CAD build for the part. Positions are in the model's coordinates, mm. A direction names the side the tool comes from. Round coordinates to 2 decimals unless told otherwise and drop trailing zeros. Order: outer loops, then holes, each group sorted by start corner. A loop starts at its lowest first (then second) coordinate and runs counter-clockwise, first axis right, second up. Notation, with made-up numbers: M 41,47 L 55,47 A18 cw 55,74 Z; hole C 41.25,40 d4. An arc over 180 degrees is marked long. Answer as a JSON object with one key per item and string values.
```python
from build123d import *
from build123d.topology import SkipClean

# Parameters (mm, degrees)
SKETCH4_R           = 9
BOSS_EXTRUDE1_DEPTH = 3
BOSS_EXTRUDE3_START = 7
SKETCH5_R           = 11.15
BOSS_EXTRUDE3_DEPTH = 7
BOSS_EXTRUDE4_START = 10
BOSS_EXTRUDE4_DEPTH = 10
BOSS_EXTRUDE5_START = 10
BOSS_EXTRUDE5_DEPTH = 10
SKETCH8_R           = 2.75
CUT_EXTRUDE2_DEPTH  = 10
SKETCH10_W          = 17
SKETCH10_H          = 20
BOSS_EXTRUDE7_DEPTH = 7
SKETCH11_W          = 8.5
SKETCH11_H          = 20
BOSS_EXTRUDE8_DEPTH = 20
SKETCH12_R          = 2.75
CUT_EXTRUDE3_DEPTH  = 20


with BuildPart() as part:
    # Sketch4 → Boss-Extrude1 (new body)
    with BuildSketch(Plane(origin=(0, 0, -7), x_dir=(-1, 0, 0), z_dir=(0, 0, -1))):
        with BuildLine():
            Line((0, 55), (0, 15))
            ThreePointArc((0, 15), (-15, 0), (0, -15))
            Line((0, -15), (0, -75))
            Line((0, -75), (17, -75))
            Line((17, -75), (17, 55))
            Line((17, 55), (0, 55))
        make_face()
        Circle(SKETCH4_R, mode=Mode.SUBTRACT)
    extrude(amount=BOSS_EXTRUDE1_DEPTH)

    # Sketch5 → Boss-Extrude3 (add)
    with BuildSketch(Plane.XY.offset(-7).offset(BOSS_EXTRUDE3_START)):
        with BuildLine():
            Line((0, -55), (0, -15))
            ThreePointArc((0, -15), (15, 0), (0, 15))
            Line((0, 15), (0, 55))
            Line((0, 55), (-17, 55))
            Line((-17, 55), (-17, -55))
            Line((-17, -55), (0, -55))
        make_face()
        Circle(SKETCH5_R, mode=Mode.SUBTRACT)
    extrude(amount=-BOSS_EXTRUDE3_DEPTH)

    # Sketch6 → Boss-Extrude4 (add)
    with SkipClean():  # the faces are left unmerged after this step: merging them gives an invalid solid
        with BuildSketch(Plane.XY.offset(BOSS_EXTRUDE4_START)):
            with BuildLine():
                Line((-8.5, 7.21612777), (-8.5, 15))
                Line((-8.5, 15), (-8.5, 55))
                Line((-8.5, 55), (-17, 55))
                Line((-17, 55), (-17, -55))
                Line((-17, -55), (-8.5, -55))
                Line((-8.5, -55), (-8.5, -16.073942755))
                Line((-8.5, -16.073942755), (-8.5, -15))
                Line((-8.5, -15), (-8.5, -7.21612777))
                ThreePointArc((-8.5, -7.21612777), (-11.15, 0), (-8.5, 7.21612777))
            make_face()
        extrude(amount=-BOSS_EXTRUDE4_DEPTH)

    # Sketch7 → Boss-Extrude5 (add)
    with SkipClean():  # the faces are left unmerged after this step: merging them gives an invalid solid
        with BuildSketch(Plane.XY.offset(10).offset(BOSS_EXTRUDE5_START)):
            with BuildLine():
                Line((-8.5, 7.21612777), (-8.5, 55))
                Line((-8.5, 55), (-17, 55))
                Line((-17, 55), (-17, -55))
                Line((-17, -55), (-8.5, -55))
                Line((-8.5, -55), (-8.5, -7.21612777))
                ThreePointArc((-8.5, -7.21612777), (-11.15, 0), (-8.5, 7.21612777))
            make_face()
        extrude(amount=-BOSS_EXTRUDE5_DEPTH)

    # Sketch8 → Cut-Extrude2 (cut)
    with SkipClean():  # the faces are left unmerged after this step: merging them gives an invalid solid
        with BuildSketch(Plane(origin=(-8.5, 0, 0), x_dir=(0, 0, -1), z_dir=(1, 0, 0))):
            with BuildLine():
                ThreePointArc((-7.25, 41.25), (-8.055456352, 43.194543648), (-10, 44))
                Line((-10, 44), (-10, 38.5))
                ThreePointArc((-10, 38.5), (-8.055456352, 39.305456352), (-7.25, 41.25))
            make_face()
            with BuildLine():
                Line((-10, 38.5), (-10, 44))
                ThreePointArc((-10, 44), (-12.75, 41.25), (-10, 38.5))
            make_face()
            with Locations((-10, 13.75)):
                Circle(SKETCH8_R)
            with Locations((-10, -13.75)):
                Circle(SKETCH8_R)
            with Locations((-10, -41.25)):
                Circle(SKETCH8_R)
        extrude(amount=-CUT_EXTRUDE2_DEPTH, mode=Mode.SUBTRACT)

    # Sketch10 → Boss-Extrude7 (add)
    with SkipClean():  # the faces are left unmerged after this step: merging them gives an invalid solid
        with BuildSketch(Plane.XY.offset(-7)):
            with Locations((-8.5, -65)):
                Rectangle(SKETCH10_W, SKETCH10_H)
        extrude(amount=BOSS_EXTRUDE7_DEPTH)

    # Sketch11 → Boss-Extrude8 (add)
    with SkipClean():  # the faces are left unmerged after this step: merging them gives an invalid solid
        with BuildSketch(Plane.XZ.offset(55)):
            with Locations((-12.75, 10)):
                Rectangle(SKETCH11_W, SKETCH11_H)
        extrude(amount=BOSS_EXTRUDE8_DEPTH)

    # Sketch12 → Cut-Extrude3 (cut)
    with SkipClean():  # the faces are left unmerged after this step: merging them gives an invalid solid
        with BuildSketch(Plane(origin=(-8.5, 0, 0), x_dir=(0, 0, -1), z_dir=(1, 0, 0))):
            with Locations(Location((-10, -65, 0), (0, 0, 90))):
                Circle(SKETCH12_R)
        extrude(amount=-CUT_EXTRUDE3_DEPTH, mode=Mode.SUBTRACT)


solid = part.part
```
Item 1: Saw through at C-C on y = -41.25. List the corners of the cut face in (x, z), and give its area (3 significant figures).
Worked answers:
{"outline": "M -17,-10 L 0,-10 L 0,0 L -8.5,0 L -8.5,7.25 L -17,7.25 Z; M -17,12.75 L -8.5,12.75 L -8.5,20 L -17,20 Z", "area": "293 mm2"}
Item 2: Drop flat-ended pins along their axis: pin 1 Ø6.5 at (y, z) = (-41.25, 10) entering from -X; pin 2 Ø6 at (y, z) = (21.5, 8) entering from +X; pin 3 Ø10 at (x, y) = (-3.5, -4.5) entering from +Z; pin 4 Ø3 at (x, y) = (9.5, -15.5) entering from +Z. Give the stop position or say it passes through.
Worked answers:
{"pin 1": "stops at x = -17", "pin 2": "stops at x = -8.5", "pin 3": "stops at z = -7", "pin 4": "passes through"}
Item 3: Saw through at A-A on z = -5.75. List the corners of the cut face in (x, y), and give its area (3 significant figures).
Worked answers:
{"outline": "M -17,-75 L 0,-75 L 0,-15 A15 ccw 0,15 L 0,55 L -17,55 Z; hole C 0,0 d22.3", "area": "2,170 mm2"}
Item 4: Two-plate mould, pull along Y, no slides. Class faces 6 (the cylindrical face through (15, 0, -5)), 7 (the cylindrical face through (-12.69, -67.747, 10.121)), 8 (the flat face through (-8.5, -41, 5)): released by +Y, released by -Y, zero draft, split by the parting line, or undercut.
Worked answers:
{"face 6": "split by the parting line", "face 7": "undercut", "face 8": "zero draft"}
Item 5: Saw through at D-D on x = -14. List the corners of the cut face in (y, z), and give its area (3 significant figures).
Worked answers:
{"outline": "M -75,-10 L 55,-10 L 55,20 L -75,20 Z; hole C -65,10 d5.5; hole C -41.25,10 d5.5; hole C -13.75,10 d5.5; hole C 13.75,10 d5.5; hole C 41.25,10 d5.5", "area": "3,780 mm2"}
Item 6: 3-axis set-ups, long thin cutter, end or side, ignore diameter. For faces 1 (the flat face through (-6, -10, 0)), 2 (the flat face through (-17, -9, 5)), 3 (the flat face through (0, -45, -5)), 4 (the flat face through (0, 35, -5)), 5 (the flat face through (-0.77, 9.14, -7)): which of +Z, -Z, +X, -X, +Y, -Y reach the whole face in a straight line?
Worked answers:
{"face 1": "+Z, +X, +Y, -Y", "face 2": "+Z, -Z, -X, +Y, -Y", "face 3": "+Z, -Z, +X, -Y", "face 4": "+Z, -Z, +X, +Y", "face 5": "+Z"}
Item 7: Wall check: line 1 along X through (y, z) = (0, -3.75); line 2 along Z through (x, y) = (-10.75, -13.75); line 3 along X through (y, z) = (-43.5, -6.25). Give the ranges that are in metal, low to high. Write a range as [from, to].
Worked answers:
{"line 1": "x = [-17, -11.15], [11.15, 15]", "line 2": "z = [-10, 7.25], [12.75, 20]", "line 3": "x = [-17, 0]"}
Item 8: Saw through at B-B on x = -6. List the corners of the cut face in (y, z), and give its area (3 significant figures).
Worked answers:
{"outline": "M -75,-10 L -6.71,-10 L -6.71,-7 L -9.4,-7 L -9.4,0 L -75,0 Z; M 6.71,-10 L 55,-10 L 55,0 L 9.4,0 L 9.4,-7 L 6.71,-7 Z", "area": "1,130 mm2"}
